Geometry check sheet. Reference: drawing and pictorial views, mm from the part's lowest x, y, z. A direction names the side the tool comes from. Coordinates: 2 decimals unless noted, no trailing zeros. Order: outer loops, then holes, each group sorted by start corner. A loop starts at its lowest first (then second) coordinate and runs counter-clockwise, first axis right, second up. Notation, with made-up numbers: M 20.5,9.5 L 70.5,9.5 A37 ccw 70.5,45.5 Z; hole C 86.5,5 d7. An arc over 180 degrees is marked long. Return JSON: item names as keys, results as strings.
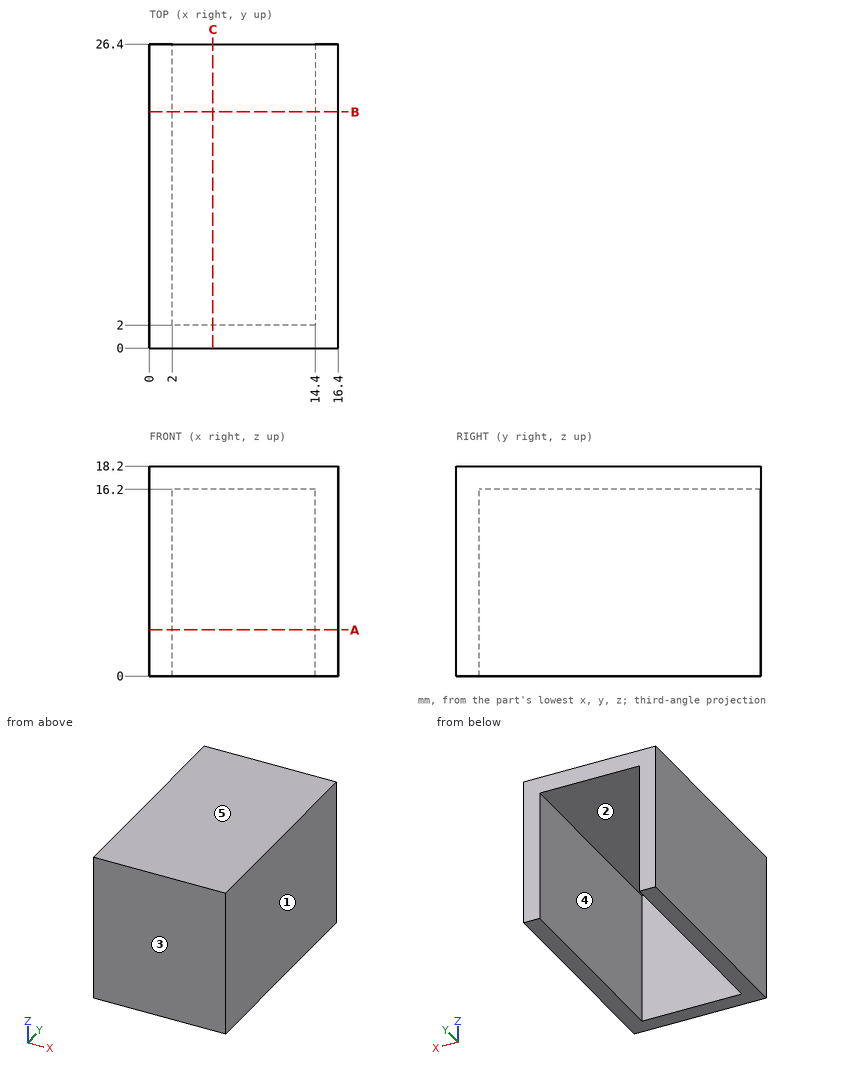
Q1. Tool access check on the marked faces 4 and 5. Record the directions out of +Z, -Z, +X, -X, +Y, -Y that give a thin tool (end or side, any length) a straight path to the whole face; none if there is none.
Values:
{"face 4": "-Z, +Y", "face 5": "+Z, +X, -X, +Y, -Y"}
Q2. Go/stop test with flat-tipped pins: pin 1 (3.5 mm diameter, centred on x = 9.5, z = 5.5, fed in from +Y); pin 2 (1.5 mm diameter, centred on x = 13, z = 6.5, fed in from -Y); pin 3 (2 mm diameter, centred on x = 7, y = 16.5, fed in from -Z). Record where each tip stops, or that it passes through.
Values:
{"pin 1": "y = 2", "pin 2": "y = 0", "pin 3": "z = 16.2"}
Q3. Material ranges on line 1 along X through (y, z) = (20, 14.25); line 2 along Y through (x, z) = (14, 12); line 3 along Z through (x, y) = (12.25, 16.75), recorded low to high.
Values:
{"line 1": "0 to 2, 14.4 to 16.4", "line 2": "0 to 2", "line 3": "16.2 to 18.2"}
Q4. Cross-section at B-B, the plane y = 20.5. Record the boundary of the cut face in (x, z).
Values:
{"outline": "M 0,0 L 2,0 L 2,16.2 L 14.4,16.2 L 14.4,0 L 16.4,0 L 16.4,18.2 L 0,18.2 Z"}
Q5. Draft check along X on the marked faces 1, 2 and 3. Enter one of: pulls with the +X half, pulls with the -X half, needs draft (parallel to the pull), parting line crosses it, or undercut.
Values:
{"face 1": "pulls with the +X half", "face 2": "undercut", "face 3": "needs draft"}
Q6. Cross-section at A-A, the plane z = 4. Record the boundary of the cut face in (x, y).
Values:
{"outline": "M 0,0 L 16.4,0 L 16.4,26.4 L 14.4,26.4 L 14.4,2 L 2,2 L 2,26.4 L 0,26.4 Z"}
Q7. Cross-section at C-C, the plane x = 5.5. Record the boundary of the cut face in (y, z), and give its area (3 significant figures).
Values:
{"outline": "M 0,0 L 2,0 L 2,16.2 L 26.4,16.2 L 26.4,18.2 L 0,18.2 Z", "area": "85.2 mm^2"}
